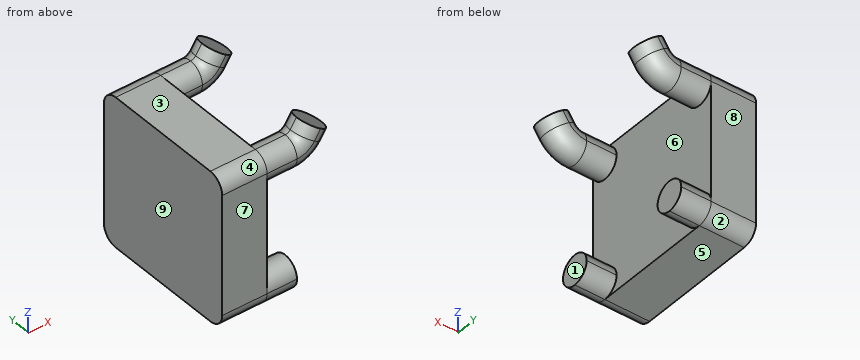
from build123d import *

# Parameters (mm, degrees)
F0_W      = 31.75
F0_H      = 31.75
F1_DEPTH  = 9.525
F10_DEPTH = 6.35
F11_R     = 3.1749


# Not quite as in the source:
# - a fillet or chamfer is up to 0.001 mm smaller than in the source, because OpenCascade refuses the exact size


with BuildPart() as f1:
    # F0 (on Right) → F1 (new body)
    with BuildSketch(Plane.YZ):
        Rectangle(F0_W, F0_H)
    extrude(amount=F1_DEPTH)

    # F6: sweep along a path in F5
    with BuildLine(Plane.XZ.offset(12.7)) as f6_path:
        Line((9.525, 9.525), (15.875, 9.525))
        ThreePointArc((15.875, 9.525), (19.4783384003, 10.4308096264), (22.225, 12.9328865162))
        Line((22.225, 12.9328865162), (23.5505334947, 14.9312034475))
    # F2 (on face) → F6 (sweep)
    with BuildSketch(Plane.YZ.offset(9.525)):
        with BuildLine():
            ThreePointArc((-15.875, 12.7), (-12.7, 9.525), (-9.525, 12.7))
            ThreePointArc((-9.525, 12.7), (-10.4549359718, 14.9450640323), (-12.7000000057, 15.875))
            ThreePointArc((-12.7000000057, 15.875), (-14.9450640323, 14.9450640282), (-15.875, 12.7))
        make_face()
    sweep(path=f6_path.line)

    # F9: F1 across plane


with BuildPart() as f1_1:
    add(f1.part)
    add(f1.part.mirror(Plane(origin=(0, 0, 15.875), x_dir=(1, 0, 0), z_dir=(0, -1, 0))))

    # F2 (on face) → F10 (join)
    with BuildSketch(Plane.YZ.offset(9.525)):
        with BuildLine():
            ThreePointArc((-9.525, -12.7), (-12.7, -9.525), (-15.875, -12.7))
            ThreePointArc((-15.875, -12.7), (-14.9450640303, -14.9450640303), (-12.7, -15.875))
            ThreePointArc((-12.7, -15.875), (-10.4549359697, -14.9450640303), (-9.525, -12.7))
        make_face()
        with BuildLine():
            ThreePointArc((12.7, -15.875), (14.9450640303, -14.9450640303), (15.875, -12.7))
            ThreePointArc((15.875, -12.7), (10.4549359697, -10.4549359697), (12.7, -15.875))
        make_face()
    extrude(amount=F10_DEPTH)

    # F11 (radius 3.175 in the source; OpenCascade refuses exactly that, so slightly less here)
    f11_edges = [f1_1.edges().sort_by_distance(p)[0] for p in [
        (4.7625, -15.875, 15.875),
        (4.7625, -15.875, -15.875),
        (4.7625, 15.875, -15.875),
        (4.7625, 15.875, 15.875),
    ]]
    fillet(f11_edges, radius=F11_R)


solid = f1_1.part
Geometry check sheet. Reference: the model listing, model coordinates, mm. Face numbers are marked on the shaded views. A direction names the side the tool comes from. Give positions to 0.01 mm unless a question says otherwise; leave off trailing zeros. Loops run counter-clockwise (first coordinate to the right, second up) from the corner with the lowest first, then second, coordinate; pieces in that order, holes last. Notation, with made-up numbers: (17.25, -13) -> (57.25, -13) arc R15 ccw to (57.25, 13) -> close; hole circle Ø11 at (41.5, 2). An arc over 180 degrees is marked (long way). Answer in a Markdown table with one row per item. Add a question column.
1) Material ranges on probe 1 along Y at (x, z) = (10.25, -12.5); probe 2 along X at (y, z) = (6, 8.5) (3 decimals); probe 3 along Z at (x, y) = (4.5, -4) (3 decimals), recorded low to high. Write a range as from..to.
2) Cross-section at A-A on x = 11.25. Record the boundary of the cut face in (y, z) (3 decimals), and give its area (3 significant figures).
3) Set-up check for the marked faces 1, 2, 3, 4 and 5: record each of +Z, -Z, +X, -X, +Y, -Y from which the full face is reachable in a straight line by a thin tool's end or side.
4) Draft check along Y on the marked faces 6, 7, 8 and 9. Enter one of: pulls with the +Y half, pulls with the -Y half, needs draft (parallel to the pull), parting line crosses it, or undercut.
5) Cross-section at B-B on z = 3.5. Record the boundary of the cut face in (x, y) (3 decimals).
6) Gauge pin test, flat ends, axial feed: P1, Ø2, axis at y = -2, z = 8.5, coming from the -X side; P2, Ø10.5, axis at x = 5, y = 4.5, coming from the +Z side (3 decimals); P3, Ø2.5, axis at y = -14, z = -15, coming from the +X side (3 decimals); P4, Ø4, axis at y = 4, z = 5.5, coming from the +X side (3 decimals). Record the tip position at first contact, or that the pin passes through.
Outcome:
| question | item | result |
|---|---|---|
| 1 | probe 1 | y = -15.87..-9.53, 9.53..15.87 |
| 1 | probe 2 | x = 0..9.525 |
| 1 | probe 3 | z = -15.875..15.875 |
| 2 | outline | circle Ø6.35 at (-12.7, -12.7); circle Ø6.35 at (-12.7, 12.7); circle Ø6.35 at (12.7, -12.7); circle Ø6.35 at (12.7, 12.7) |
| 2 | area | 127 mm^2 |
| 3 | face 1 | -Z, +X, +Y, -Y |
| 3 | face 2 | -Z, +X, -X, +Y |
| 3 | face 3 | +Z, -X, +Y, -Y |
| 3 | face 4 | +Z, -X, -Y |
| 3 | face 5 | -Z, +X, -X, +Y, -Y |
| 4 | face 6 | undercut |
| 4 | face 7 | pulls with the -Y half |
| 4 | face 8 | pulls with the +Y half |
| 4 | face 9 | needs draft |
| 5 | outline | (0, -15.875) -> (9.525, -15.875) -> (9.525, 15.875) -> (0, 15.875) -> close |
| 6 | P1 | stops at x = 0 |
| 6 | P2 | stops at z = 15.875 |
| 6 | P3 | stops at x = 15.875 |
| 6 | P4 | stops at x = 9.525 |
